```python
from build123d import *

# Parameters (mm, degrees)
SKETCH1_W           = 18
SKETCH1_H           = 12
BOSS_EXTRUDE1_DEPTH = 1
SKETCH2_R           = 1.25
BOSS_EXTRUDE2_DEPTH = 8
SKETCH3_W           = 18
SKETCH3_H           = 12
BOSS_EXTRUDE3_DEPTH = 1
BOSS_EXTRUDE4_DEPTH = 15
SKETCH5_R           = 2.5
SKETCH5_R_2         = 0.5
BOSS_EXTRUDE5_DEPTH = 1
SKETCH6_W           = 0.5
SKETCH6_H           = 1.5
BOSS_EXTRUDE6_DEPTH = 2.5
BOSS_EXTRUDE7_DEPTH = 8
SKETCH8_W           = 0.2
SKETCH8_H           = 0.1
CUT_EXTRUDE1_DEPTH  = 35.208916966


with BuildPart() as part:
    # Sketch1 → Boss-Extrude1 (new body)
    with BuildSketch(Plane(origin=(0, 0, 0), x_dir=(1, 0, 0), z_dir=(0, 1, 0))):
        Rectangle(SKETCH1_W, SKETCH1_H)
    extrude(amount=BOSS_EXTRUDE1_DEPTH)

    # Sketch2 → Boss-Extrude2 (add)
    with BuildSketch(Plane(origin=(0, 1, 0), x_dir=(1, 0, 0), z_dir=(0, 1, 0))):
        with Locations(Location((7.5, 4.5, 0), (0, 0, 90))):
            Circle(SKETCH2_R)
        with Locations(Location((7.5, -4.5, 0), (0, 0, 90))):
            Circle(SKETCH2_R)
    extrude(amount=BOSS_EXTRUDE2_DEPTH)

    # Sketch3 → Boss-Extrude3 (add)
    with BuildSketch(Plane(origin=(0, 9, 0), x_dir=(1, 0, 0), z_dir=(0, 1, 0))):
        Rectangle(SKETCH3_W, SKETCH3_H)
    extrude(amount=BOSS_EXTRUDE3_DEPTH)

    # Sketch4 → Boss-Extrude4 (add)
    with BuildSketch(Plane.ZY.offset(9)):
        with BuildLine():
            Line((-3.75, 0), (3.75, 0))
            ThreePointArc((3.75, 0), (5.406152949, 1.984423525), (6, 4.5))
            Line((6, 4.5), (6, 5.5))
            ThreePointArc((6, 5.5), (5.406152949, 8.015576475), (3.75, 10))
            Line((3.75, 10), (-3.75, 10))
            ThreePointArc((-3.75, 10), (-5.406152949, 8.015576475), (-6, 5.5))
            Line((-6, 5.5), (-6, 4.5))
            ThreePointArc((-6, 4.5), (-5.406152949, 1.984423525), (-3.75, 0))
        make_face()
    extrude(amount=BOSS_EXTRUDE4_DEPTH)

    # Sketch5 → Boss-Extrude5 (add)
    with BuildSketch(Plane.ZY.offset(24)):
        with Locations((0, 5)):
            Circle(SKETCH5_R)
        with Locations((0, 5)):
            Circle(SKETCH5_R_2, mode=Mode.SUBTRACT)
    extrude(amount=BOSS_EXTRUDE5_DEPTH)

    # Sketch6 → Boss-Extrude6 (add)
    with BuildSketch(Plane.ZY.offset(24)):
        with Locations((-3.25, 5)):
            Rectangle(SKETCH6_W, SKETCH6_H)
        with Locations((3.25, 5)):
            Rectangle(SKETCH6_W, SKETCH6_H)
    extrude(amount=BOSS_EXTRUDE6_DEPTH)

    # Sketch7 → Boss-Extrude7 (add)
    with BuildSketch(Plane(origin=(0, 10, 0), x_dir=(1, 0, 0), z_dir=(0, 1, 0))):
        with BuildLine():
            Line((5.75, -0.829156198), (5.75, 0.829156198))
            ThreePointArc((5.75, 0.829156198), (3, 0), (5.75, -0.829156198))
        make_face()
    extrude(amount=BOSS_EXTRUDE7_DEPTH)

    # Sketch8 → Cut-Extrude1 (cut, through all)
    with BuildSketch(Plane.XY.offset(6)):
        with Locations((-9.1, 9.95)):
            Rectangle(SKETCH8_W, SKETCH8_H)
        with Locations((-9.1, 0.05)):
            Rectangle(SKETCH8_W, SKETCH8_H)
    extrude(amount=-CUT_EXTRUDE1_DEPTH, mode=Mode.SUBTRACT)


solid = part.part
```
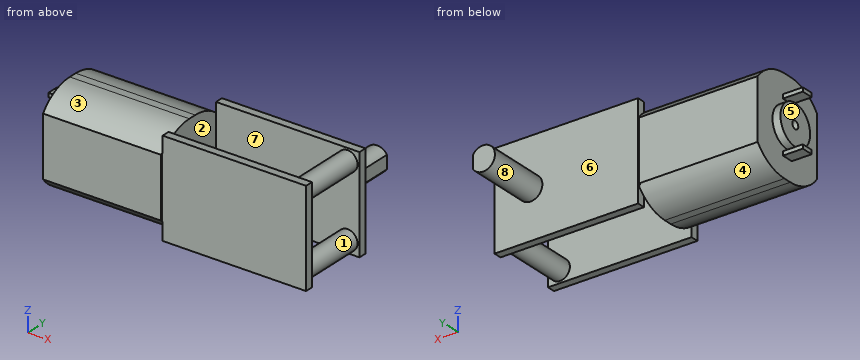
Read the model definition and answer for the solid it produces. Units are mm, in the model's axes. Face numbers are marked on the shaded views. A direction names the side the tool comes from. Give positions to 0.01 mm unless a question says otherwise; leave off trailing zeros. Order: outer loops, then holes, each group sorted by start corner. A loop starts at its lowest first (then second) coordinate and runs counter-clockwise, first axis right, second up. Notation, with made-up numbers: (28.25, 48) -> (35.25, 48) arc R26 ccw to (35.25, 77) -> close; hole circle Ø1 at (-4, 51). An arc over 180 degrees is marked (long way). One line per item, written item: value. Start each with the question number.
(1) The part is cut by section D-D (z = -2). Determine the outline of the cut face in (x, y), and give its area (3 significant figures).
(2) The part is cut by section C-C (x = 7.5). Determine the outline of the cut face in (y, z).
(3) For a pull along Y with two mould halves and no side action, classify the marked faces 6, 7 and 8 as released by +Y, released by -Y, zero draft, split by the parting line, or undercut.
(4) A tool of negligible diameter and unlimited length cuts with its end or side. For the marked faces 1, 2, 3, 4 and 5, from which of +Z, -Z, +X, -X, +Y, -Y can it reach the whole face along a straight path? Write none if from no direction.
(5) Flat-ended cylindrical pins translate along their axes: P1, Ø10, axis at x = -20, y = 9, coming from the -Z side; P2, Ø1.1, axis at y = 9.5, z = 0.5, coming from the -X side; P3, Ø5.5, axis at y = 4, z = 0, coming from the -X side; P4, Ø2, axis at x = -13.5, y = 10, coming from the +Z side. Find the tip coordinate at first contact, or state that the pin passes through.
(6) Straight lines are drawn through the part: L1, parallel to Y at x = -24.55, z = 0; L2, parallel to Y at x = -3.5, z = 1.5; L3, parallel to Y at x = -10, z = 2.75. For each, find the intervals that lie inside material, in ascending order.
(7) The part is cut by section A-A (y = 5). Determine the outline of the cut face in (x, z), and give its area (3 significant figures).
(8) The part is cut by section B-B (x = -6.5). Determine the outline of the cut face in (y, z), and give its area (3 significant figures).
Taken from the geometry:
1. outline: (-25, 3.5) -> (-24, 3.5) -> (-24, 0) -> (-9.2, 0) -> (-9.2, 0.1) -> (-9, 0.1) -> (-9, 0) -> (9, 0) -> (9, 1) -> (-9, 1) -> (-9, 9) -> (9, 9) -> (9, 10) -> (-9, 10) -> (-9, 9.9) -> (-9.2, 9.9) -> (-9.2, 10) -> (-24, 10) -> (-24, 6.5) -> (-25, 6.5) -> close
1. area: 189 mm^2
2. outline: (0, -6) -> (1, -6) -> (1, -5.75) -> (9, -5.75) -> (9, -6) -> (10, -6) -> (10, 6) -> (9, 6) -> (9, 5.75) -> (1, 5.75) -> (1, 6) -> (0, 6) -> close; hole (1, -3.25) -> (9, -3.25) -> (9, 3.25) -> (1, 3.25) -> close
3. face 6: released by +Y
3. face 7: undercut
3. face 8: zero draft
4. face 1: none
4. face 2: +Z, -Z
4. face 3: +Z, -X, -Y
4. face 4: -Z, -X, +Y
4. face 5: -X, +Y, -Y
5. P1: z = -6
5. P2: x = -24
5. P3: x = -25
5. P4: z = 4.78
6. L1: 2.5 to 4.5, 5.5 to 7.5
6. L2: 0 to 1, 9 to 10
6. L3: 0 to 10
7. outline: (-26.5, -3.5) -> (-24, -3.5) -> (-24, -6) -> (-9, -6) -> (-9, 6) -> (-24, 6) -> (-24, 3.5) -> (-26.5, 3.5) -> (-26.5, 3) -> (-24, 3) -> (-24, 2.5) -> (-25, 2.5) -> (-25, 0.5) -> (-24, 0.5) -> (-24, -0.5) -> (-25, -0.5) -> (-25, -2.5) -> (-24, -2.5) -> (-24, -3) -> (-26.5, -3) -> close; circle Ø2.5 at (7.5, -4.5); circle Ø2.5 at (7.5, 4.5)
7. area: 196 mm^2
8. outline: (0, -6) -> (1, -6) -> (1, 6) -> (0, 6) -> close; (9, -6) -> (10, -6) -> (10, 6) -> (9, 6) -> close
8. area: 24.0 mm^2
